Design review of the part shown in the three views and the two pictorial views. Dimensions are in mm from the part's minimum x, y and z. Coordinates: 2 decimals unless noted, no trailing zeros. Loops run counter-clockwise (first coordinate to the right, second up) from the corner with the lowest first, then second, coordinate; pieces in that order, holes last. Notation, with made-up numbers: M -26.5,-29.5 L 0.5,-29.5 A35 ccw 0.5,9.5 Z; hole C 28,89.25 d4. An arc over 180 degrees is marked long. Use one line per item in the form item = value.
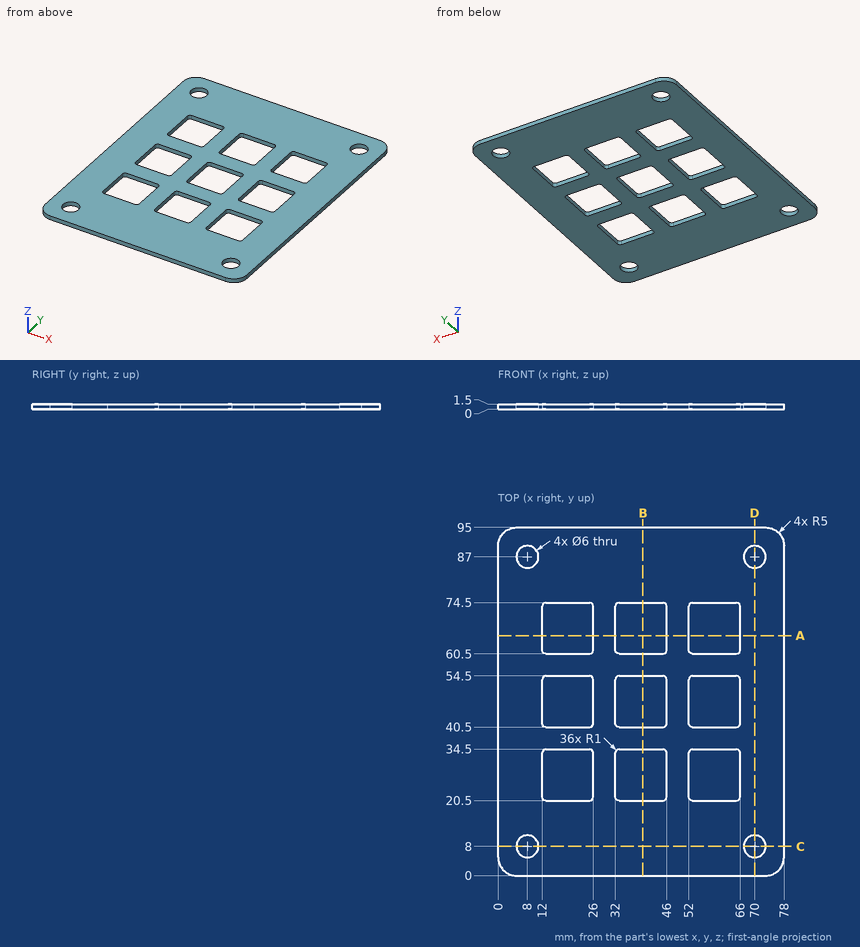
1. Add section A-A (y = 65.5). State the section outline as (x, z) points, then the cut area to 3 significant figures.
Response values:
outline = M 0,0 L 12,0 L 12,1.5 L 0,1.5 Z; M 26,0 L 32,0 L 32,1.5 L 26,1.5 Z; M 46,0 L 52,0 L 52,1.5 L 46,1.5 Z; M 66,0 L 78,0 L 78,1.5 L 66,1.5 Z
area = 54.0 mm^2
2. Add section C-C (y = 8). State the section outline as (x, z) points.
Response values:
outline = M 0,0 L 5,0 L 5,1.5 L 0,1.5 Z; M 11,0 L 67,0 L 67,1.5 L 11,1.5 Z; M 73,0 L 78,0 L 78,1.5 L 73,1.5 Z
3. Add section D-D (x = 70). State the section outline as (y, z) points.
Response values:
outline = M 0,0 L 5,0 L 5,1.5 L 0,1.5 Z; M 11,0 L 84,0 L 84,1.5 L 11,1.5 Z; M 90,0 L 95,0 L 95,1.5 L 90,1.5 Z
4. Add section B-B (x = 39.5). State the section outline as (y, z) points, then the cut area to 3 significant figures.
Response values:
outline = M 0,0 L 20.5,0 L 20.5,1.5 L 0,1.5 Z; M 34.5,0 L 40.5,0 L 40.5,1.5 L 34.5,1.5 Z; M 54.5,0 L 60.5,0 L 60.5,1.5 L 54.5,1.5 Z; M 74.5,0 L 95,0 L 95,1.5 L 74.5,1.5 Z
area = 79.5 mm^2
5. Wall thickness on line 1 along Y through (x, z) = (70, 1.05); line 2 along X through (y, z) = (31, 1.05); line 3 along Y through (x, z) = (23.5, 0.15): over which ranges is each line inside the solid? List them lowest first. Write a range as from..to.
Response values:
line_1 = 0..5, 11..84, 90..95
line_2 = 0..12, 26..32, 46..52, 66..78
line_3 = 0..20.5, 34.5..40.5, 54.5..60.5, 74.5..95
